The listing builds one solid part. Answer for the finished solid, in the listing's coordinates (mm). A direction names the side the tool comes from. Round coordinates to 2 decimals unless told otherwise and drop trailing zeros. Loops run counter-clockwise (first coordinate to the right, second up) from the corner with the lowest first, then second, coordinate; pieces in that order, holes last. Notation, with made-up numbers: (-24.5, -21.5) - (21.5, -21.5) arc R32 cw to (21.5, 9.5) - close; hole circle Ø1 at (71, 62). An arc over 180 degrees is marked (long way). Write item = value, one per line. Start each with the question number.
1) Section B-B, the plane x = 9.25 is taken. Determine the outline of the cut face in (y, z), and give its area (3 significant figures).
2) Given pin 1 Ø1.7 at (x, z) = (15, 0) entering from +Y; pin 2 Ø1 at (x, z) = (12, 2.5) entering from +Y; pin 3 Ø4 at (x, y) = (9.5, 1.5) entering from -Z, each flat-ended and moving along its own axis, determine where each tip first touches the part or whether it passes through.
3) Straight lines are drawn through the part: line 1 along X through (y, z) = (-1.4, 0); line 2 along Z through (x, y) = (14.25, 0); line 3 along Z through (x, y) = (15, -1.95). For each, find the intervals that lie inside material, in ascending order.
4) A tool of negligible diameter and unlimited length cuts with its end or side. For faces 1 (the flat face through (18, 0, 0)), 2 (the cylindrical face through (9.85, -0.65, -2.93)), from which of +Z, -Z, +X, -X, +Y, -Y can it reach the whole face along a straight path? Write none if from no direction.
5) Section C-C, the plane x = 15 is taken. Determine the outline of the cut face in (y, z), and give its area (3 significant figures).
6) Section A-A, the plane z = 0 is taken. Determine the outline of the cut face in (x, y), and give its area (3 significant figures).
from build123d import *

# Parameters (mm, degrees)
CHAMFER1_R      = 0.5
SKETCH2_R       = 1.07
HOLE_DEPTH      = 6
HOLE_DEPTH_BACK = 6.0000001


with BuildPart() as part:
    # Sketch1 → BaseBody (revolve)
    with BuildSketch(Plane.XY):
        with BuildLine():
            Line((18, 0), (0, 0))
            Line((0, 0), (0, 4))
            ThreePointArc((0, 4), (1, 5), (2, 4))
            Line((2, 4), (2, 3))
            Line((2, 3), (17, 3))
            Line((17, 3), (18, 2.422649731))
            Line((18, 2.422649731), (18, 0))
        make_face()
    revolve(axis=Axis((-19.830028721, 0, 0), (1, 0, 0)))

    # Chamfer1
    chamfer1_edges = [part.edges().sort_by_distance(p)[0] for p in [
        (2, -3, 0),
    ]]
    fillet(chamfer1_edges, radius=CHAMFER1_R)

    # Sketch2 → Hole (cut, two sides)
    with BuildSketch(Plane(origin=(0, 0, 0), x_dir=(1, 0, 0), z_dir=(0, 1, 0))) as hole_sk:
        with Locations((15, 0)):
            Circle(SKETCH2_R)
    extrude(amount=HOLE_DEPTH, mode=Mode.SUBTRACT)
    extrude(hole_sk.sketch, amount=-HOLE_DEPTH_BACK, mode=Mode.SUBTRACT)


solid = part.part
Geometry check:
q1.outline = circle Ø6 at (0, 0)
q1.area = 28.3 mm2
q2.pin_1 = through
q2.pin_2 = 2.24
q2.pin_3 = -3
q3.line_1 = 0 to 13.93, 16.07 to 18
q3.line_2 = -3 to -0.76, 0.76 to 3
q3.line_3 = -2.28 to -1.07, 1.07 to 2.28
q4.face_1 = +Z, -Z, +X, +Y, -Y
q4.face_2 = +X
q5.outline = (-2.8, -1.07) arc R3 ccw to (2.8, -1.07) - close; (-2.8, 1.07) - (2.8, 1.07) arc R3 ccw to start
q5.area = 15.7 mm2
q6.outline = (0, -4) arc R1 ccw to (2, -4) - (2, -3.5) arc R0.5 cw to (2.5, -3) - (13.93, -3) - (13.93, 3) - (2.5, 3) arc R0.5 cw to (2, 3.5) - (2, 4) arc R1 ccw to (0, 4) - close; (16.07, -3) - (17, -3) - (18, -2.42) - (18, 2.42) - (17, 3) - (16.07, 3) - close
q6.area = 102 mm2
